Can you work these out from the drawing? Everything is in mm from the part's minimum corner. Round coordinates to 2 decimals unless told otherwise and drop trailing zeros. Order: outer loops, then holes, each group sorted by start corner. A loop starts at its lowest first (then second) coordinate and runs counter-clockwise, first axis right, second up. Notation, with made-up numbers: M 23,26 L 36,26 A29 ccw 36,50 Z; hole C 6.25,-10.75 d6. An arc over 180 degrees is marked long. Use one line per item in the form item = value. Start each with the question number.
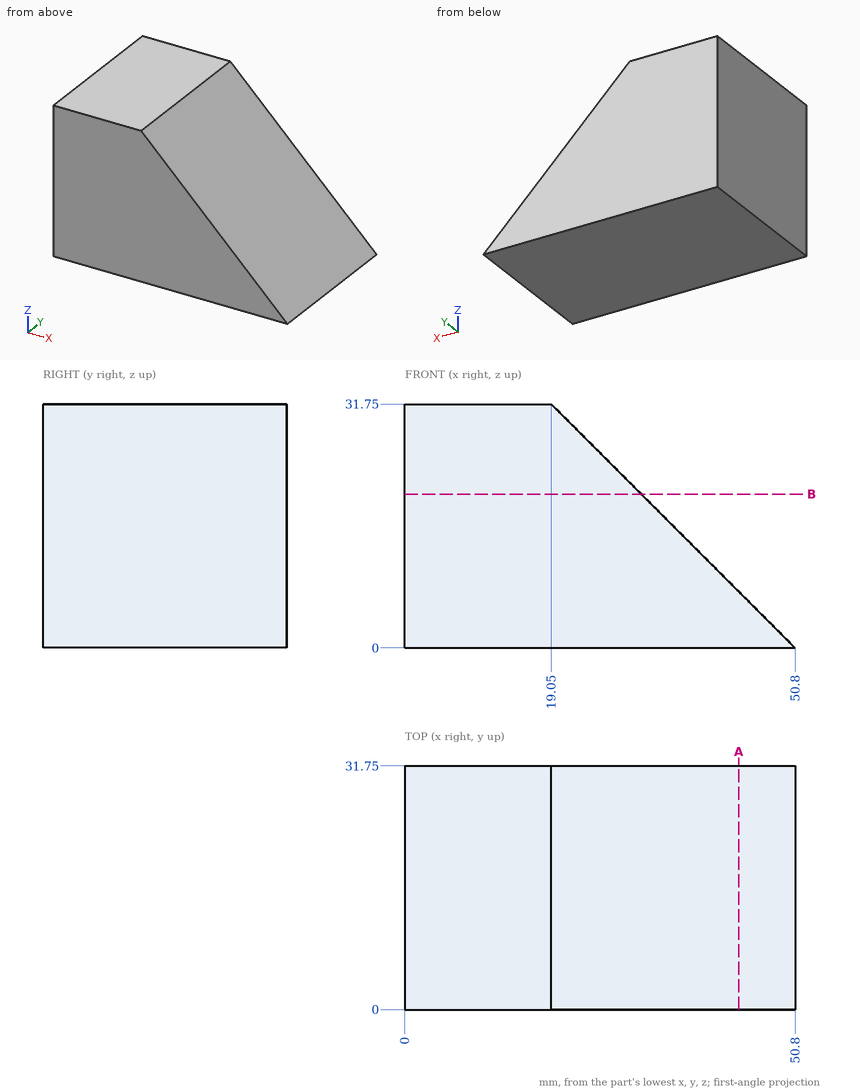
1) If we section it at A-A on x = 43.5: Write out the boundary of the cut face in (y, z).
2) Will these pins go through, and if not, where does the flat tip stop? pin 1 Ø8 at (x, y) = (34.5, 18) entering from +Z; pin 2 Ø1.5 at (x, y) = (29, 10) entering from +Z; pin 3 Ø4 at (x, z) = (41, 13) entering from +Y.
3) If we section it at B-B on z = 20: Write out the boundary of the cut face in (x, y).
4) If I drill on line 1 (X direction, y = 16.5, z = 26); line 2 (X direction, y = 12.5, z = 2.5); line 3 (Z direction, x = 47.5, y = 27), over which ranges is the centre line in solid material (lowest first)?
Completed:
q1.outline = M 0,0 L 31.75,0 L 31.75,7.3 L 0,7.3 Z
q2.pin_1 = 20.3
q2.pin_2 = 22.55
q2.pin_3 = through
q3.outline = M 0,0 L 30.8,0 L 30.8,31.75 L 0,31.75 Z
q4.line_1 = 0 to 24.8
q4.line_2 = 0 to 48.3
q4.line_3 = 0 to 3.3
